```python
from build123d import *

# Parameters (mm, degrees)
SKETCH1_R                = 50
BOSS_EXTRUDE1_DEPTH      = 50
BOSS_EXTRUDE2_REACH      = 218.16
BOSS_EXTRUDE2_END_RADIUS = 65
SKETCH2_R                = 45


with BuildPart() as part:
    # Sketch1 → Boss-Extrude1 (new, symmetric)
    with BuildSketch(Plane.XY):
        with BuildLine():
            Line((-80, -40), (-80, 40))
            Line((-80, 40), (-17.368072784, 62.636650994))
            ThreePointArc((-17.368072784, 62.636650994), (65, 0), (-17.368072784, -62.636650994))
            Line((-17.368072784, -62.636650994), (-80, -40))
        make_face()
        with Locations(Location((0, 0, 0), (0, 0, 180))):
            Circle(SKETCH1_R, mode=Mode.SUBTRACT)
    extrude(amount=BOSS_EXTRUDE1_DEPTH, both=True)

    # Boss-Extrude2: up to this cylinder (the profile starts outside it)
    boss_extrude2_end = Plane(origin=(0, 0, 0), z_dir=(0, 0, -1)) * Cylinder(BOSS_EXTRUDE2_END_RADIUS, 567.32, mode=Mode.PRIVATE)
    # Sketch2 → Boss-Extrude2 (add, up to the surface)
    with BuildSketch(Plane(origin=(120, 0, 0), x_dir=(0, 0, -1), z_dir=(1, 0, 0)), mode=Mode.PRIVATE) as boss_extrude2_sk1:
        Circle(SKETCH2_R)
    boss_extrude2_tool1 = extrude(boss_extrude2_sk1.sketch, amount=-BOSS_EXTRUDE2_REACH, mode=Mode.PRIVATE) - boss_extrude2_end
    add(boss_extrude2_tool1.solids().sort_by_distance((120, 0, 0))[0])

    # Sketch3 → Revolve1 (revolve)
    with BuildSketch(Plane.XY, mode=Mode.PRIVATE) as revolve1_sk:
        Polygon((120, 0), (120, -20), (134, -20), (134, -25), (149, -25), (149, -17.556833969), (158, -13.197935025), (158, -7.068196984), (195, 0), align=None)
    revolve(revolve1_sk.sketch.rotate(Axis((353.949576891, 0, 0), (-1, 0, 0)), 270), axis=Axis((353.949576891, 0, 0), (-1, 0, 0)))


solid = part.part
```
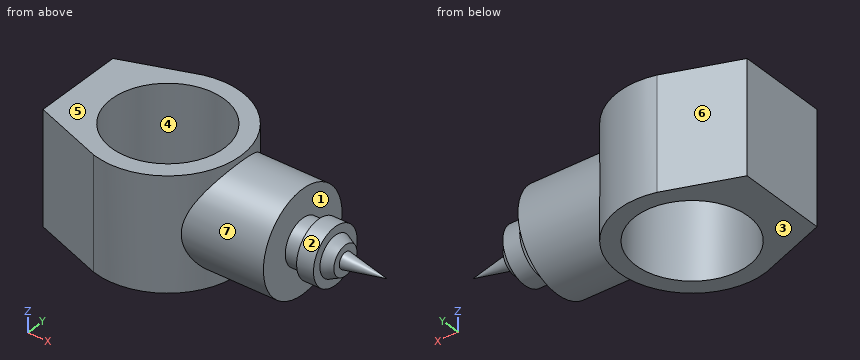
Check sheet for the modelled part. Datum: model origin and axes. Units: mm. Face numbers are marked on the shaded views. A direction names the side the tool comes from. Coordinates: 2 decimals unless noted, no trailing zeros. Order: outer loops, then holes, each group sorted by start corner. A loop starts at its lowest first (then second) coordinate and runs counter-clockwise, first axis right, second up. Notation, with made-up numbers: M -2,17 L 38,17 A25 cw 38,42 Z; hole C 47.25,-14 d6. An arc over 180 degrees is marked long. One line per question, with ' | ' between items. Start each with the question number.
Item 1: Mould release check, pull along Y, two halves, no side actions. Record for the marked faces 4, 5, 6 and 7: pulls with the +Y half, pulls with the -Y half, needs draft (parallel to the pull), parting line crosses it, or undercut.
Item 2: Sectioned sample at A-A on x = 0. Record the cut outline in (y, z), and give its area (3 significant figures).
Item 3: Sectioned sample at C-C on x = 59. Record the cut outline in (y, z).
Item 4: Sectioned sample at D-D on y = 35. Record the cut outline in (x, z), and give its area (3 significant figures).
Item 5: Sectioned sample at B-B on y = -35.5. Record the cut outline in (x, z), and give its area (3 significant figures).
Item 6: Material ranges on line 1 (Y direction, x = 0, z = 21); line 2 (X direction, y = 16, z = -31.5); line 3 (Y direction, x = -33, z = 16), recorded low to high.
Item 7: Gauge pin test, flat ends, axial feed: P1, Ø5, axis at y = -21.5, z = -7.5, coming from the +X side; P2, Ø10, axis at x = 11.5, z = 21.5, coming from the -Y side; P3, Ø6, axis at x = -34, z = 22, coming from the +Y side; P4, Ø10, axis at x = 68, y = 8.5, coming from the +Z side. Record the tip position at first contact, or that the pin passes through.
Item 8: Access from +Z, -Z, +X, -X, +Y, -Y to the whole of each face (thin tool, end or side, straight path). Record for the marked faces 1, 2 and 3.
Answer below:
1) face 4: undercut | face 5: needs draft | face 6: pulls with the +Y half | face 7: parting line crosses it
2) outline: M -65,-50 L -50,-50 L -50,50 L -65,50 Z; M 50,-50 L 65,-50 L 65,50 L 50,50 Z | area: 3,000 mm^2
3) outline: M -27.28,-50 L 27.28,-50 L 27.28,-35.79 A45 ccw 27.28,35.79 L 27.28,50 L -27.28,50 L -27.28,35.79 A45 ccw -27.28,-35.79 Z
4) outline: M -80,-50 L -35.71,-50 L -35.71,50 L -80,50 Z; M 35.71,-50 L 54.77,-50 L 54.77,-28.28 L 120,-28.28 L 120,28.28 L 54.77,28.28 L 54.77,50 L 35.71,50 Z | area: 10,000 mm^2
5) outline: M -80,-50 L -35.21,-50 L -35.21,50 L -80,50 Z; M 35.21,-50 L 54.45,-50 L 54.45,-27.65 L 120,-27.65 L 120,27.65 L 54.45,27.65 L 54.45,50 L 35.21,50 Z | area: 10,000 mm^2
6) line 1: y = -65 to -50, 50 to 65 | line 2: x = -80 to -47.37, 47.37 to 120 | line 3: y = -56.99 to -37.56, 37.56 to 56.99
7) P1: stops at x = 149 | P2: stops at y = -64.67 | P3: stops at y = 57.71 | P4: stops at z = 50
8) face 1: none | face 2: +X | face 3: -Z, +X, -X, +Y, -Y
